Geometry check sheet. Reference: the model listing, model coordinates, mm. Face numbers are marked on the shaded views. A direction names the side the tool comes from. Coordinates: 2 decimals unless noted, no trailing zeros. Order: outer loops, then holes, each group sorted by start corner. A loop starts at its lowest first (then second) coordinate and runs counter-clockwise, first axis right, second up. Notation, with made-up numbers: (-24, -26) - (21, -26) arc R15 cw to (21, -4) - close; hole circle Ø10 at (71.5, 58.25). An arc over 180 degrees is marked (long way). Return JSON: item names as keys, results as strings. Group by question number.
Item 1: Scan lines: probe 1 along Y at (x, z) = (-1.5, 7.25); probe 2 along X at (y, z) = (9, 2.5); probe 3 along Z at (x, y) = (5, 4). Record each from-to range of solid material in increasing order.
Item 2: Section check C-C on x = -4.5. Enter the section's corners in (y, z), then the cut area to 3 significant figures.
Item 3: Section check B-B on y = 2.5. Enter the section's corners in (x, z), then the cut area to 3 significant figures.
Item 4: Gauge pin test, flat ends, axial feed: pin 1 (0.6 mm diameter, centred on x = 4.5, y = 6, fed in from +Z); pin 2 (1 mm diameter, centred on x = 14.5, y = -1.5, fed in from +Z); pin 3 (0.8 mm diameter, centred on x = -13, y = -4.5, fed in from +Z). Record the tip position at first contact, or that the pin passes through.
Item 5: Draft check along Y on the marked faces 1, 2, 3 and 4. Enter one of: pulls with the +Y half, pulls with the -Y half, needs draft (parallel to the pull), parting line crosses it, or undercut.
Item 6: Section check A-A on z = 8.75. Enter the section's corners in (x, y).
Item 7: Tool access check on the marked faces 5 and 6. Record the directions out of +Z, -Z, +X, -X, +Y, -Y that give a thin tool (end or side, any length) a straight path to the whole face; none if there is none.
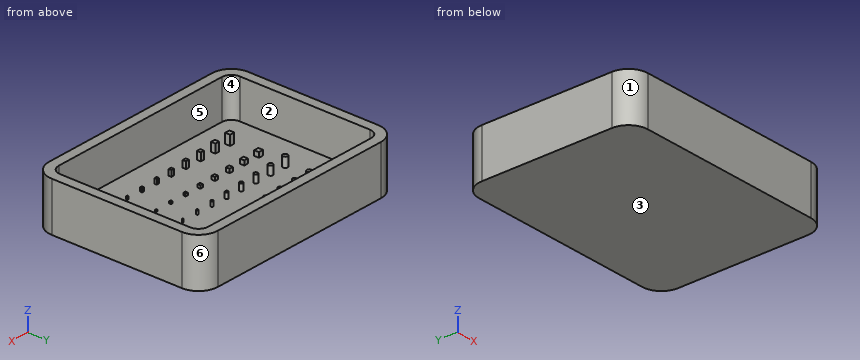
from build123d import *

# Parameters (mm, degrees)
SKETCH1_W            = 47
SKETCH1_H            = 35
BOSS_EXTRUDE1_DEPTH  = 10
FILLET1_R            = 4
SHELL1_T             = -2
SKETCH2_R            = 0.5
BOSS_EXTRUDE6_DEPTH  = 1
SKETCH3_R            = 0.45
BOSS_EXTRUDE7_DEPTH  = 0.9
SKETCH4_R            = 0.4
BOSS_EXTRUDE8_DEPTH  = 0.8
SKETCH5_R            = 0.35
BOSS_EXTRUDE9_DEPTH  = 0.7
SKETCH6_R            = 0.3
BOSS_EXTRUDE10_DEPTH = 0.6
SKETCH7_R            = 0.25
BOSS_EXTRUDE11_DEPTH = 0.5
SKETCH8_R            = 0.2
BOSS_EXTRUDE12_DEPTH = 0.4
SKETCH9_R            = 0.15
BOSS_EXTRUDE13_DEPTH = 0.3
SKETCH10_R           = 0.5
BOSS_EXTRUDE14_DEPTH = 2
SKETCH11_R           = 0.45
BOSS_EXTRUDE15_DEPTH = 1.8
SKETCH12_R           = 0.4
BOSS_EXTRUDE16_DEPTH = 1.6
SKETCH13_R           = 0.35
BOSS_EXTRUDE17_DEPTH = 1.4
SKETCH14_R           = 0.3
BOSS_EXTRUDE18_DEPTH = 1.2
SKETCH15_R           = 0.25
BOSS_EXTRUDE19_DEPTH = 1
SKETCH16_R           = 0.2
BOSS_EXTRUDE20_DEPTH = 0.8
SKETCH17_R           = 0.15
BOSS_EXTRUDE21_DEPTH = 0.6
SKETCH18_W           = 1
SKETCH18_H           = 1
BOSS_EXTRUDE22_DEPTH = 1
SKETCH20_W           = 0.9
SKETCH20_H           = 0.9
BOSS_EXTRUDE23_DEPTH = 0.9
SKETCH21_W           = 0.8
SKETCH21_H           = 0.8
BOSS_EXTRUDE24_DEPTH = 0.8
SKETCH22_W           = 0.7
SKETCH22_H           = 0.7
BOSS_EXTRUDE25_DEPTH = 0.7
SKETCH23_W           = 0.6
SKETCH23_H           = 0.6
BOSS_EXTRUDE26_DEPTH = 0.6
SKETCH24_W           = 0.5
SKETCH24_H           = 0.5
BOSS_EXTRUDE27_DEPTH = 0.5
SKETCH25_W           = 0.4
SKETCH25_H           = 0.4
BOSS_EXTRUDE28_DEPTH = 0.4
SKETCH26_W           = 0.3
SKETCH26_H           = 0.3
BOSS_EXTRUDE29_DEPTH = 0.3
SKETCH27_W           = 1
SKETCH27_H           = 1
BOSS_EXTRUDE30_DEPTH = 2
SKETCH28_W           = 0.9
SKETCH28_H           = 0.9
BOSS_EXTRUDE31_DEPTH = 1.8
SKETCH29_W           = 0.8
SKETCH29_H           = 0.8
BOSS_EXTRUDE32_DEPTH = 1.6
SKETCH30_W           = 0.7
SKETCH30_H           = 0.7
BOSS_EXTRUDE33_DEPTH = 1.4
SKETCH31_W           = 0.6
SKETCH31_H           = 0.6
BOSS_EXTRUDE34_DEPTH = 1.2
SKETCH32_W           = 0.5
SKETCH32_H           = 0.5
BOSS_EXTRUDE35_DEPTH = 1
SKETCH33_W           = 0.4
SKETCH33_H           = 0.4
BOSS_EXTRUDE36_DEPTH = 0.8
SKETCH34_W           = 0.3
SKETCH34_H           = 0.3
BOSS_EXTRUDE37_DEPTH = 0.6


with BuildPart() as part:
    # Sketch1 → Boss-Extrude1 (new body)
    with BuildSketch(Plane.XY):
        with Locations((2.008287293, -0.759668508)):
            Rectangle(SKETCH1_W, SKETCH1_H)
    extrude(amount=BOSS_EXTRUDE1_DEPTH)

    # Fillet1
    fillet1_edges = [part.edges().sort_by_distance(p)[0] for p in [
        (-21.491712707, 16.740331492, 5),
        (25.508287293, 16.740331492, 5),
        (25.508287293, -18.259668508, 5),
        (-21.491712707, -18.259668508, 5),
    ]]
    fillet(fillet1_edges, radius=FILLET1_R)

    # Shell1
    shell1_openings = [part.faces().sort_by_distance(p)[0] for p in [
        (2.008287293, -0.759668508, 10),
    ]]
    offset(amount=SHELL1_T, openings=shell1_openings, kind=Kind.INTERSECTION)

    # Sketch2 → Boss-Extrude6 (add)
    with BuildSketch(Plane.XY.offset(2)):
        with Locations((-12.824656071, 5.939639856)):
            Circle(SKETCH2_R)
    extrude(amount=BOSS_EXTRUDE6_DEPTH)

    # Sketch3 → Boss-Extrude7 (add)
    with BuildSketch(Plane.XY.offset(2)):
        with Locations((-9.324656071, 5.939639856)):
            Circle(SKETCH3_R)
    extrude(amount=BOSS_EXTRUDE7_DEPTH)

    # Sketch4 → Boss-Extrude8 (add)
    with BuildSketch(Plane.XY.offset(2)):
        with Locations((-5.824656071, 5.939639856)):
            Circle(SKETCH4_R)
    extrude(amount=BOSS_EXTRUDE8_DEPTH)

    # Sketch5 → Boss-Extrude9 (add)
    with BuildSketch(Plane.XY.offset(2)):
        with Locations((-2.324656071, 5.939639856)):
            Circle(SKETCH5_R)
    extrude(amount=BOSS_EXTRUDE9_DEPTH)

    # Sketch6 → Boss-Extrude10 (add)
    with BuildSketch(Plane.XY.offset(2)):
        with Locations((1.175343929, 5.939639856)):
            Circle(SKETCH6_R)
    extrude(amount=BOSS_EXTRUDE10_DEPTH)

    # Sketch7 → Boss-Extrude11 (add)
    with BuildSketch(Plane.XY.offset(2)):
        with Locations((4.675343929, 5.939639856)):
            Circle(SKETCH7_R)
    extrude(amount=BOSS_EXTRUDE11_DEPTH)

    # Sketch8 → Boss-Extrude12 (add)
    with BuildSketch(Plane.XY.offset(2)):
        with Locations((8.175343929, 5.939639856)):
            Circle(SKETCH8_R)
    extrude(amount=BOSS_EXTRUDE12_DEPTH)

    # Sketch9 → Boss-Extrude13 (add)
    with BuildSketch(Plane.XY.offset(2)):
        with Locations((11.675343929, 5.939639856)):
            Circle(SKETCH9_R)
    extrude(amount=BOSS_EXTRUDE13_DEPTH)

    # Sketch10 → Boss-Extrude14 (add)
    with BuildSketch(Plane.XY.offset(2)):
        with Locations((-12.824656071, 0.939639856)):
            Circle(SKETCH10_R)
    extrude(amount=BOSS_EXTRUDE14_DEPTH)

    # Sketch11 → Boss-Extrude15 (add)
    with BuildSketch(Plane.XY.offset(2)):
        with Locations((-9.324656071, 0.931713012)):
            Circle(SKETCH11_R)
    extrude(amount=BOSS_EXTRUDE15_DEPTH)

    # Sketch12 → Boss-Extrude16 (add)
    with BuildSketch(Plane.XY.offset(2)):
        with Locations((-5.824656071, 0.931713012)):
            Circle(SKETCH12_R)
    extrude(amount=BOSS_EXTRUDE16_DEPTH)

    # Sketch13 → Boss-Extrude17 (add)
    with BuildSketch(Plane.XY.offset(2)):
        with Locations((-2.324656071, 0.931713012)):
            Circle(SKETCH13_R)
    extrude(amount=BOSS_EXTRUDE17_DEPTH)

    # Sketch14 → Boss-Extrude18 (add)
    with BuildSketch(Plane.XY.offset(2)):
        with Locations((1.175343929, 0.931713012)):
            Circle(SKETCH14_R)
    extrude(amount=BOSS_EXTRUDE18_DEPTH)

    # Sketch15 → Boss-Extrude19 (add)
    with BuildSketch(Plane.XY.offset(2)):
        with Locations((4.675343929, 0.931713012)):
            Circle(SKETCH15_R)
    extrude(amount=BOSS_EXTRUDE19_DEPTH)

    # Sketch16 → Boss-Extrude20 (add)
    with BuildSketch(Plane.XY.offset(2)):
        with Locations((8.175343929, 0.931713012)):
            Circle(SKETCH16_R)
    extrude(amount=BOSS_EXTRUDE20_DEPTH)

    # Sketch17 → Boss-Extrude21 (add)
    with BuildSketch(Plane.XY.offset(2)):
        with Locations((11.675343929, 0.931713012)):
            Circle(SKETCH17_R)
    extrude(amount=BOSS_EXTRUDE21_DEPTH)

    # Sketch18 → Boss-Extrude22 (add)
    with BuildSketch(Plane.XY.offset(2)):
        with Locations((-12.821712707, -4.560360144)):
            Rectangle(SKETCH18_W, SKETCH18_H)
    extrude(amount=BOSS_EXTRUDE22_DEPTH)

    # Sketch20 → Boss-Extrude23 (add)
    with BuildSketch(Plane.XY.offset(2)):
        with Locations((-9.324656071, -4.560360144)):
            Rectangle(SKETCH20_W, SKETCH20_H)
    extrude(amount=BOSS_EXTRUDE23_DEPTH)

    # Sketch21 → Boss-Extrude24 (add)
    with BuildSketch(Plane.XY.offset(2)):
        with Locations((-5.824656071, -4.560360144)):
            Rectangle(SKETCH21_W, SKETCH21_H)
    extrude(amount=BOSS_EXTRUDE24_DEPTH)

    # Sketch22 → Boss-Extrude25 (add)
    with BuildSketch(Plane.XY.offset(2)):
        with Locations((-2.324656071, -4.560360144)):
            Rectangle(SKETCH22_W, SKETCH22_H)
    extrude(amount=BOSS_EXTRUDE25_DEPTH)

    # Sketch23 → Boss-Extrude26 (add)
    with BuildSketch(Plane.XY.offset(2)):
        with Locations((1.175343929, -4.560360144)):
            Rectangle(SKETCH23_W, SKETCH23_H)
    extrude(amount=BOSS_EXTRUDE26_DEPTH)

    # Sketch24 → Boss-Extrude27 (add)
    with BuildSketch(Plane.XY.offset(2)):
        with Locations((4.675343929, -4.560360144)):
            Rectangle(SKETCH24_W, SKETCH24_H)
    extrude(amount=BOSS_EXTRUDE27_DEPTH)

    # Sketch25 → Boss-Extrude28 (add)
    with BuildSketch(Plane.XY.offset(2)):
        with Locations((8.175343929, -4.560360144)):
            Rectangle(SKETCH25_W, SKETCH25_H)
    extrude(amount=BOSS_EXTRUDE28_DEPTH)

    # Sketch26 → Boss-Extrude29 (add)
    with BuildSketch(Plane.XY.offset(2)):
        with Locations((11.675343929, -4.560360144)):
            Rectangle(SKETCH26_W, SKETCH26_H)
    extrude(amount=BOSS_EXTRUDE29_DEPTH)

    # Sketch27 → Boss-Extrude30 (add)
    with BuildSketch(Plane.XY.offset(2)):
        with Locations((-12.821712707, -10.560360144)):
            Rectangle(SKETCH27_W, SKETCH27_H)
    extrude(amount=BOSS_EXTRUDE30_DEPTH)

    # Sketch28 → Boss-Extrude31 (add)
    with BuildSketch(Plane.XY.offset(2)):
        with Locations((-9.324656071, -10.560360144)):
            Rectangle(SKETCH28_W, SKETCH28_H)
    extrude(amount=BOSS_EXTRUDE31_DEPTH)

    # Sketch29 → Boss-Extrude32 (add)
    with BuildSketch(Plane.XY.offset(2)):
        with Locations((-5.824656071, -10.560360144)):
            Rectangle(SKETCH29_W, SKETCH29_H)
    extrude(amount=BOSS_EXTRUDE32_DEPTH)

    # Sketch30 → Boss-Extrude33 (add)
    with BuildSketch(Plane.XY.offset(2)):
        with Locations((-2.324656071, -10.560360144)):
            Rectangle(SKETCH30_W, SKETCH30_H)
    extrude(amount=BOSS_EXTRUDE33_DEPTH)

    # Sketch31 → Boss-Extrude34 (add)
    with BuildSketch(Plane.XY.offset(2)):
        with Locations((1.175343929, -10.560360144)):
            Rectangle(SKETCH31_W, SKETCH31_H)
    extrude(amount=BOSS_EXTRUDE34_DEPTH)

    # Sketch32 → Boss-Extrude35 (add)
    with BuildSketch(Plane.XY.offset(2)):
        with Locations((4.675343929, -10.560360144)):
            Rectangle(SKETCH32_W, SKETCH32_H)
    extrude(amount=BOSS_EXTRUDE35_DEPTH)

    # Sketch33 → Boss-Extrude36 (add)
    with BuildSketch(Plane.XY.offset(2)):
        with Locations((8.175343929, -10.560360144)):
            Rectangle(SKETCH33_W, SKETCH33_H)
    extrude(amount=BOSS_EXTRUDE36_DEPTH)

    # Sketch34 → Boss-Extrude37 (add)
    with BuildSketch(Plane.XY.offset(2)):
        with Locations((11.675343929, -10.560360144)):
            Rectangle(SKETCH34_W, SKETCH34_H)
    extrude(amount=BOSS_EXTRUDE37_DEPTH)


solid = part.part
Computed:
{
 "1": {"probe 1": "y = -18.26 to -16.26, 14.74 to 16.74", "probe 2": "x = -21.49 to -19.49, 23.51 to 25.51", "probe 3": "z = 0 to 2"},
 "2": {"outline": "(-18.26, 0) - (16.74, 0) - (16.74, 10) - (14.74, 10) - (14.74, 2) - (-16.26, 2) - (-16.26, 10) - (-18.26, 10) - close", "area": "102 mm²"},
 "3": {"outline": "(-21.49, 0) - (25.51, 0) - (25.51, 10) - (23.51, 10) - (23.51, 2) - (-19.49, 2) - (-19.49, 10) - (-21.49, 10) - close", "area": "126 mm²"},
 "4": {"pin 1": "stops at z = 2.5", "pin 2": "stops at z = 2", "pin 3": "stops at z = 3"},
 "5": {"face 1": "pulls with the -Y half", "face 2": "undercut", "face 3": "needs draft", "face 4": "undercut"},
 "6": {"outline": "(-21.49, -14.26) arc R4 ccw to (-17.49, -18.26) - (21.51, -18.26) arc R4 ccw to (25.51, -14.26) - (25.51, 12.74) arc R4 ccw to (21.51, 16.74) - (-17.49, 16.74) arc R4 ccw to (-21.49, 12.74) - close; hole (-19.49, -14.26) arc R2 ccw to (-17.49, -16.26) - (21.51, -16.26) arc R2 ccw to (23.51, -14.26) - (23.51, 12.74) arc R2 ccw to (21.51, 14.74) - (-17.49, 14.74) arc R2 ccw to (-19.49, 12.74) - close"},
 "7": {"face 5": "+Z", "face 6": "+Z, -Z, +X, +Y"}
}
